from build123d import *

# Parameters (mm, degrees)
F0_W      = 30
F0_H      = 85
F1_DEPTH  = 6
F2_R      = 3.5
F3_DEPTH  = 4
F4_R      = 2.1
F5_DEPTH  = 25
F6_R      = 3.5
F7_DEPTH  = 4
F8_R      = 2.1
F9_DEPTH  = 25
F11_R     = 1.25
F12_DEPTH = 10
F10_R     = 1.25
F13_DEPTH = 10


with BuildPart() as f1:
    # F0 (on Top) → F1 (new body)
    with BuildSketch(Plane.XY):
        with Locations((15, 42.5)):
            Rectangle(F0_W, F0_H)
    extrude(amount=F1_DEPTH)

    # F2 (on face) → F3 (cut)
    with BuildSketch(Plane.XY.offset(6)):
        with Locations((15, 80)):
            Circle(F2_R)
    extrude(amount=-F3_DEPTH, mode=Mode.SUBTRACT)

    # F4 (on face) → F5 (cut)
    with BuildSketch(Plane.XY.offset(2)):
        with Locations((15, 80)):
            Circle(F4_R)
    extrude(amount=-F5_DEPTH, mode=Mode.SUBTRACT)

    # F6 (on face) → F7 (cut)
    with BuildSketch(Plane.XY.offset(6)):
        with Locations((14.787185, 6.874469)):
            Circle(F6_R)
    extrude(amount=-F7_DEPTH, mode=Mode.SUBTRACT)

    # F8 (on face) → F9 (cut)
    with BuildSketch(Plane.XY.offset(2)):
        with Locations((14.787185, 6.874469)):
            Circle(F8_R)
    extrude(amount=-F9_DEPTH, mode=Mode.SUBTRACT)

    # F11 (on face) → F12 (cut)
    with BuildSketch(Plane(origin=(0, 0, 0), x_dir=(0, -1, 0), z_dir=(-1, 0, 0))):
        with Locations((-73, 3)):
            Circle(F11_R)
    extrude(amount=-F12_DEPTH, mode=Mode.SUBTRACT)

    # F10 (on face) → F13 (cut)
    with BuildSketch(Plane(origin=(0, 0, 0), x_dir=(0, -1, 0), z_dir=(-1, 0, 0))):
        with Locations((-3, 3)):
            Circle(F10_R)
    extrude(amount=-F13_DEPTH, mode=Mode.SUBTRACT)


solid = f1.part
Could you check a few things on this model? Use its own coordinates, in mm. A direction names the side the tool comes from. Give positions to 0.01 mm unless a question says otherwise; leave off trailing zeros. Order: outer loops, then holes, each group sorted by start corner. A loop starts at its lowest first (then second) coordinate and runs counter-clockwise, first axis right, second up. Notation, with made-up numbers: (61.25, 87) -> (111.25, 87) arc R20 cw to (111.25, 92) -> close; hole circle Ø2 at (37, 59). An arc over 180 degrees is marked (long way). Return JSON: item names as keys, results as strings.
1. Thinking about a two-plate mould opening in X: for faces 1 (the flat face through (14.7, 4.6, 2)), 2 (the flat face through (15, 43, 6)), 3 (the flat face through (30, 42, 3)), 4 (the flat face through (10, 73, 3)), which applies, pulls with the +X half, pulls with the -X half, needs draft (parallel to the pull), parting line crosses it, or undercut?
Answer list:
{"face 1": "undercut", "face 2": "needs draft", "face 3": "pulls with the +X half", "face 4": "pulls with the -X half"}
2. Imagine slicing it at B-B on x = 15. List the corners of the cut face in (y, z) for me.
Answer list:
{"outline": "(0, 0) -> (4.79, 0) -> (4.79, 2) -> (3.38, 2) -> (3.38, 6) -> (0, 6) -> close; (8.96, 0) -> (77.9, 0) -> (77.9, 2) -> (76.5, 2) -> (76.5, 6) -> (10.37, 6) -> (10.37, 2) -> (8.96, 2) -> close; (82.1, 0) -> (85, 0) -> (85, 6) -> (83.5, 6) -> (83.5, 2) -> (82.1, 2) -> close"}
3. Imagine slicing it at D-D on x = 3.5. List the corners of the cut face in (y, z) for me.
Answer list:
{"outline": "(0, 0) -> (85, 0) -> (85, 6) -> (0, 6) -> close; hole circle Ø2.5 at (3, 3); hole circle Ø2.5 at (73, 3)"}
4. I need wall thicknesses on line 1 (Y direction, x = 15, z = 4.5); line 2 (Y direction, x = 4.5, z = 3.1); line 3 (Z direction, x = 2.5, y = 73). Which ranges of each line are inside material? Lowest first, please. Write a range as from..to.
Answer list:
{"line 1": "y = 0..3.38, 10.37..76.5, 83.5..85", "line 2": "y = 0..1.75, 4.25..71.75, 74.25..85", "line 3": "z = 0..1.75, 4.25..6"}
5. Imagine slicing it at C-C on z = 3. List the corners of the cut face in (x, y) for me.
Answer list:
{"outline": "(0, 0) -> (30, 0) -> (30, 85) -> (0, 85) -> (0, 74.25) -> (10, 74.25) -> (10, 71.75) -> (0, 71.75) -> (0, 4.25) -> (10, 4.25) -> (10, 1.75) -> (0, 1.75) -> close; hole circle Ø7 at (14.79, 6.87); hole circle Ø7 at (15, 80)"}
6. For pin 1 Ø4 at (x, y) = (15, 80) entering from +Z; pin 2 Ø2 at (x, y) = (14.5, 78.5) entering from +Z; pin 3 Ø1.2 at (y, z) = (3, 2.5) entering from -X, each with a flat end and sliding along its axis, tell me the tip position at first contact or that it passes through.
Answer list:
{"pin 1": "passes through", "pin 2": "stops at z = 2", "pin 3": "stops at x = 10"}
7. On a 3-axis mill with a long thin cutter (end or side, diameter ignored), from which of +Z, -Z, +X, -X, +Y, -Y can I reach the whole of each face in a straight line? I mean faces 5 (the cylindrical face through (4.93, 71.81, 3.38)), 6 (the cylindrical face through (14.241, 76.583, 4.028)), 7 (the cylindrical face through (14.54, 77.95, 1.01)). Say none if no direction works.
Answer list:
{"face 5": "-X", "face 6": "+Z", "face 7": "+Z, -Z"}
8. Imagine slicing it at A-A on y = 80. List the corners of the cut face in (x, z) for me.
Answer list:
{"outline": "(0, 0) -> (12.9, 0) -> (12.9, 2) -> (11.5, 2) -> (11.5, 6) -> (0, 6) -> close; (17.1, 0) -> (30, 0) -> (30, 6) -> (18.5, 6) -> (18.5, 2) -> (17.1, 2) -> close"}
